The drawing under review shows one solid part. Ordinate dimensions are in mm from its lowest x, y, z. Coordinates: 2 decimals unless noted, no trailing zeros. Order: outer loops, then holes, each group sorted by start corner. A loop starts at its lowest first (then second) coordinate and runs counter-clockwise, first axis right, second up.
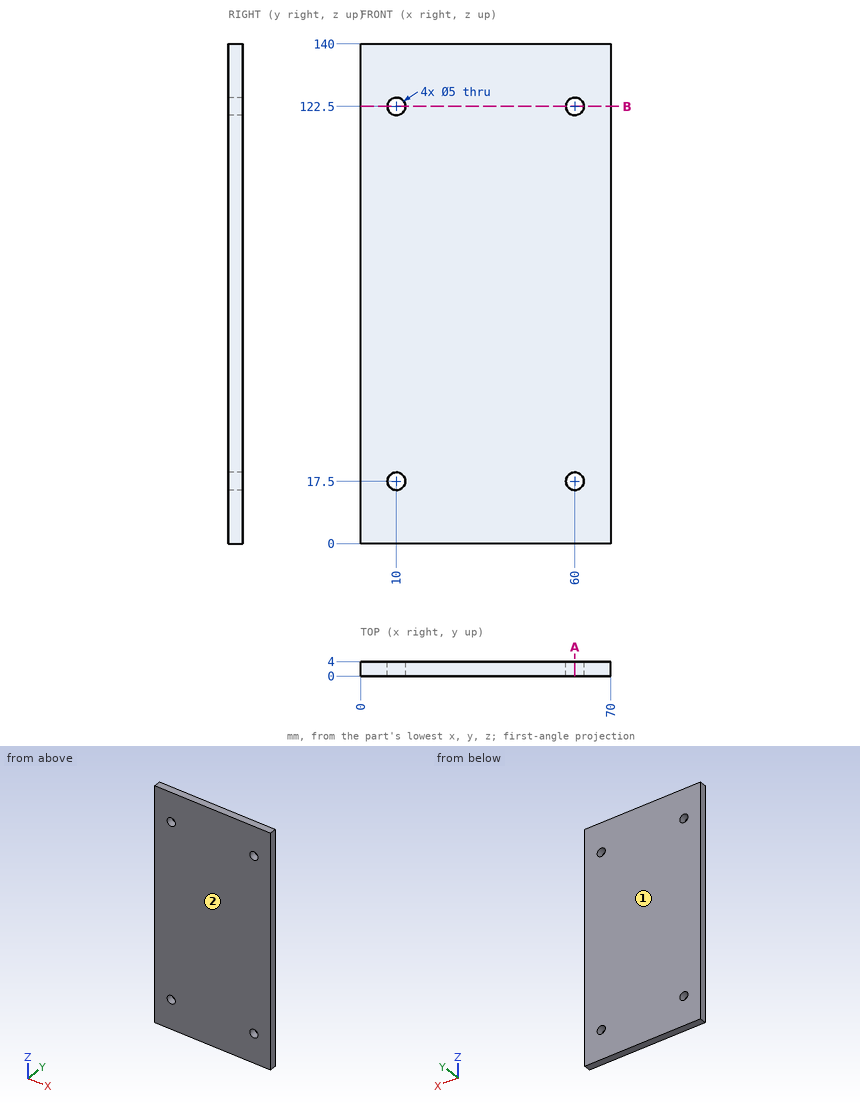
1. Mouldability with a two-part tool opening along Y and no side actions: class the marked faces 1 and 2 as pulls with the +Y half, pulls with the -Y half, needs draft (parallel to the pull), parting line crosses it, or undercut.
2. Add section A-A (x = 60). Give the boundary of the cut face in (y, z).
3. Insertion check: pin 1 (1 mm diameter, centred on x = 17.5, y = 1, fed in from -Z); pin 2 (4 mm diameter, centred on x = 10, z = 17.5, fed in from -Y). Each pin has a flat end and moves straight along its axis. Give the tip position at first contact, or say it passes through.
4. To check wall thickness, follow line 1 (X direction, y = 0.9, z = 122.5); line 2 (Z direction, x = 60, y = 1.65); line 3 (Z direction, x = 8.5, y = 1.25). State the ranges of each line that lie inside material, in increasing order.
5. Add section B-B (z = 122.5). Give the boundary of the cut face in (x, y), and give its area (3 significant figures).
Solution:
1. face 1: pulls with the +Y half
1. face 2: pulls with the -Y half
2. outline: (0, 0) - (4, 0) - (4, 15) - (0, 15) - close; (0, 20) - (4, 20) - (4, 120) - (0, 120) - close; (0, 125) - (4, 125) - (4, 140) - (0, 140) - close
3. pin 1: stops at z = 0
3. pin 2: passes through
4. line 1: x = 0 to 7.5, 12.5 to 57.5, 62.5 to 70
4. line 2: z = 0 to 15, 20 to 120, 125 to 140
4. line 3: z = 0 to 15.5, 19.5 to 120.5, 124.5 to 140
5. outline: (0, 0) - (7.5, 0) - (7.5, 4) - (0, 4) - close; (12.5, 0) - (57.5, 0) - (57.5, 4) - (12.5, 4) - close; (62.5, 0) - (70, 0) - (70, 4) - (62.5, 4) - close
5. area: 240 mm2
